Input: part model. Units: mm. Frame: model coordinates. Face numbers are marked on the shaded views. A direction names the side the tool comes from. Coordinates: 2 decimals unless noted, no trailing zeros. Order: outer loops, then holes, each group sorted by start corner. A loop starts at its lowest first (then second) coordinate and runs counter-clockwise, first axis right, second up. Notation, with made-up numbers: M -6,23.25 L 44,23.25 A16 cw 44,39.25 Z; hole C 0.5,75 d2. An arc over 180 degrees is marked long. One line per item, written item: value.
```python
from build123d import *

# Parameters (mm, degrees)
SKETCH1_R           = 30
BOSS_EXTRUDE1_DEPTH = 15
SKETCH2_R           = 10
BOSS_EXTRUDE2_DEPTH = 9
SKETCH3_R           = 3.25
CUT_EXTRUDE1_DEPTH  = 25
FILLET1_R           = 3
SKETCH8_R           = 3.05
CUT_EXTRUDE3_DEPTH  = 16
CUT_EXTRUDE4_DEPTH  = 5.2
SKETCH9_R           = 6
CUT_EXTRUDE5_DEPTH  = 5.5
CUT_EXTRUDE6_DEPTH  = 5.5
FILLET2_R           = 2


with BuildPart() as part:
    # Sketch1 → Boss-Extrude1 (new body)
    with BuildSketch(Plane.XY):
        Circle(SKETCH1_R)
    extrude(amount=BOSS_EXTRUDE1_DEPTH)

    # Sketch2 → Boss-Extrude2 (add)
    with BuildSketch(Plane.XY.offset(15)):
        Circle(SKETCH2_R)
    extrude(amount=BOSS_EXTRUDE2_DEPTH)

    # Sketch3 → Cut-Extrude1 (cut, through all)
    with BuildSketch(Plane.XY.offset(24)):
        Circle(SKETCH3_R)
    extrude(amount=-CUT_EXTRUDE1_DEPTH, mode=Mode.SUBTRACT)

    # Fillet1
    fillet1_edges = [part.edges().sort_by_distance(p)[0] for p in [
        (-3.25, 0, 0),
        (-30, 0, 0),
        (-30, 0, 15),
    ]]
    fillet(fillet1_edges, radius=FILLET1_R)

    # Sketch8 → Cut-Extrude3 (cut, through all)
    with BuildSketch(Plane.XY.offset(15)):
        with Locations((-18, 0)):
            Circle(SKETCH8_R)
    extrude(amount=-CUT_EXTRUDE3_DEPTH, mode=Mode.SUBTRACT)

    # Sketch7 → Cut-Extrude4 (cut)
    with BuildSketch(Plane.XY.offset(15)):
        Polygon((-23.1, 2.944486373), (-23.1, -2.944486373), (-18, -5.888972746), (-12.9, -2.944486373), (-12.9, 2.944486373), (-18, 5.888972746), align=None)
    extrude(amount=-CUT_EXTRUDE4_DEPTH, mode=Mode.SUBTRACT)

    # Sketch9 → Cut-Extrude5 (cut)
    with BuildSketch(Plane.XY.offset(24)):
        Circle(SKETCH9_R)
    extrude(amount=-CUT_EXTRUDE5_DEPTH, mode=Mode.SUBTRACT)

    # Sketch10 → Cut-Extrude6 (cut)
    with BuildSketch(Plane.XY.offset(18.5)):
        Polygon((5.773502692, 0), (2.886751346, 5), (-2.886751346, 5), (-5.773502692, 0), (-2.886751346, -5), (2.886751346, -5), align=None)
    extrude(amount=-CUT_EXTRUDE6_DEPTH, mode=Mode.SUBTRACT)

    # Fillet2
    fillet2_edges = [part.edges().sort_by_distance(p)[0] for p in [
        (-10, 0, 15),
    ]]
    fillet(fillet2_edges, radius=FILLET2_R)


solid = part.part
```
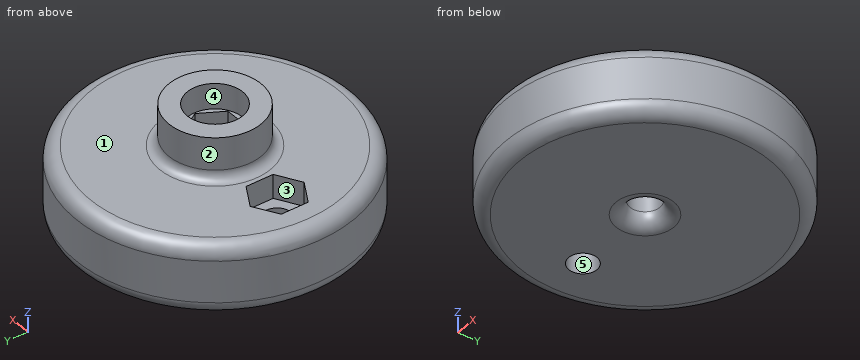
(1) Ray query, line 1 (Y direction, x = 0, z = 6.5); line 2 (Y direction, x = 0, z = 19.9); line 3 (Z direction, x = -21, y = 5). Return the intervals inside material, ascending. Write a range as from..to.
Data:
line 1: y = -30..-3.25, 3.25..30
line 2: y = -10..-6, 6..10
line 3: z = 0..15
(2) First-contact query: pin 1 (12 mm diameter, centred on y = -16.5, z = 14.5, fed in from +X); pin 2 (3 mm diameter, centred on x = -0.5, z = 8, fed in from -Y); pin 3 (1.6 mm diameter, centred on x = 1, z = 17, fed in from -Y). Flat tips, straight axial feed; report the tip coordinate or a pass-through.
Data:
pin 1: stops at x = 27.93
pin 2: stops at y = -30
pin 3: stops at y = -10.13
(3) Cut plane B-B on z = 19.5. Output: boundary loops of the cut face in (x, y).
Data:
outline: C 0,0 d20; hole C 0,0 d12
(4) Access query for the marked faces 4 and 5. Directions: +Z, -Z, +X, -X, +Y, -Y. A direction counts if a zero-diameter tool reaches every point of the face in a straight line with its end or side. Return the directions, or none.
Data:
face 4: +Z
face 5: +Z, -Z
(5) Cut plane A-A on x = 0. Output: boundary loops of the cut face in (y, z), plus the area to 3 significant figures.
Data:
outline: M -30,3 A3 ccw -27,0 L -6.25,0 A3 ccw -3.25,3 L -3.25,13 L -5,13 L -5,18.5 L -6,18.5 L -6,24 L -10,24 L -10,17 A2 cw -12,15 L -27,15 A3 ccw -30,12 Z; M 3.25,3 A3 ccw 6.25,0 L 27,0 A3 ccw 30,3 L 30,12 A3 ccw 27,15 L 12,15 A2 cw 10,17 L 10,24 L 6,24 L 6,18.5 L 5,18.5 L 5,13 L 3.25,13 Z
area: 865 mm2
(6) Cut plane C-C on z = 1.5. Output: boundary loops of the cut face in (x, y).
Data:
outline: C 0,0 d59.2; hole C -18,0 d6.1; hole C 0,0 d7.3
(7) Draft query along X for the marked faces 1, 2 and 3. Return one class per face: released by +X, released by -X, zero draft, split by the parting line, or undercut.
Data:
face 1: zero draft
face 2: split by the parting line
face 3: undercut
